Answer from the drawing. Dimensions are ordinates in mm from the lowest x, y and z of the part. Coordinates: 2 decimals unless noted, no trailing zeros. Loops run counter-clockwise (first coordinate to the right, second up) from the corner with the lowest first, then second, coordinate; pieces in that order, holes last.
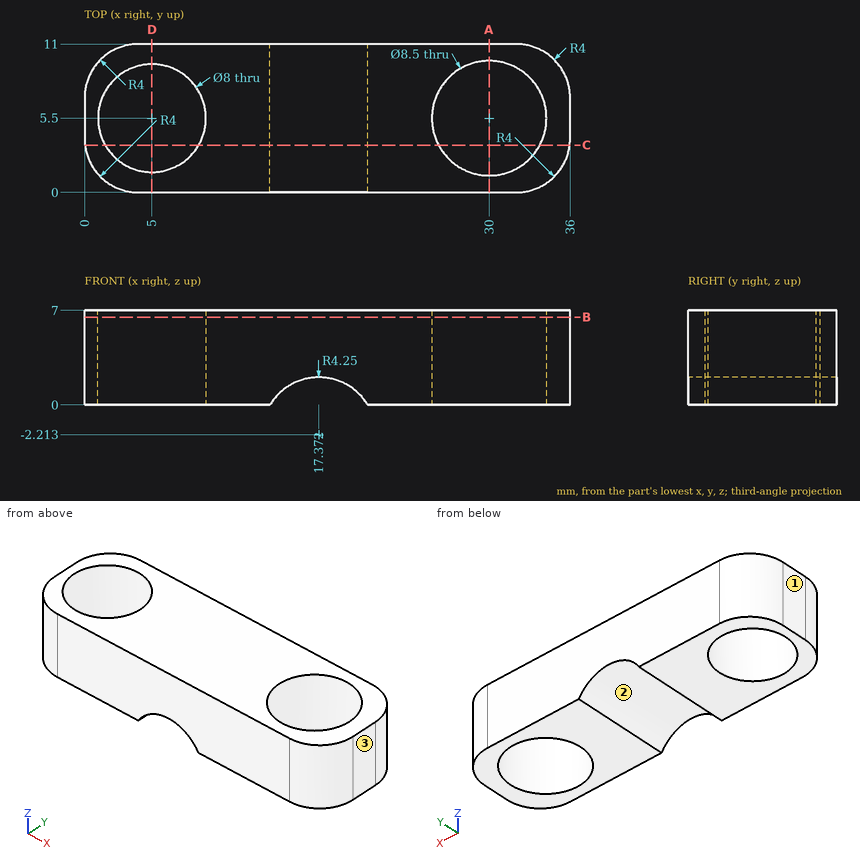
Item 1: Given pin 1 (4 mm diameter, centred on y = 1.5, z = 3.5, fed in from -X), flat-ended and moving along its own axis, determine where the tip first touches the part or whether it passes through.
Numbers:
pin 1: stops at x = 0.03
Item 2: Determine the mould class of the marked faces 1, 2 and 3 for opening direction X: released by +X, released by -X, zero draft, split by the parting line, or undercut.
Numbers:
face 1: released by -X
face 2: undercut
face 3: released by +X
Item 3: A cutting plane is placed at A-A on x = 30. Determine the outline of the cut face in (y, z).
Numbers:
outline: (0, 0) - (1.25, 0) - (1.25, 7) - (0, 7) - close; (9.75, 0) - (11, 0) - (11, 7) - (9.75, 7) - close
Item 4: A cutting plane is placed at B-B on z = 6.5. Determine the outline of the cut face in (x, y).
Numbers:
outline: (0, 4) arc R4 ccw to (4, 0) - (32, 0) arc R4 ccw to (36, 4) - (36, 7) arc R4 ccw to (32, 11) - (4, 11) arc R4 ccw to (0, 7) - close; hole circle Ø8 at (5, 5.5); hole circle Ø8.5 at (30, 5.5)
Item 5: Find the intervals of material crossed by line 1 along X through (y, z) = (5.75, 5); line 2 along Y through (x, z) = (30, 3.25); line 3 along Y through (x, z) = (5, 5), in increasing order.
Numbers:
line 1: x = 0 to 1.01, 8.99 to 25.76, 34.24 to 36
line 2: y = 0 to 1.25, 9.75 to 11
line 3: y = 0 to 1.5, 9.5 to 11
Item 6: A cutting plane is placed at D-D on x = 5. Determine the outline of the cut face in (y, z), then the cut area to 3 significant figures.
Numbers:
outline: (0, 0) - (1.5, 0) - (1.5, 7) - (0, 7) - close; (9.5, 0) - (11, 0) - (11, 7) - (9.5, 7) - close
area: 21.0 mm2
Item 7: A cutting plane is placed at C-C on y = 3.5. Determine the outline of the cut face in (x, z), then the cut area to 3 significant figures.
Numbers:
outline: (0.03, 0) - (1.54, 0) - (1.54, 7) - (0.03, 7) - close; (8.46, 0) - (13.74, 0) arc R4.25 cw to (21, 0) - (26.25, 0) - (26.25, 7) - (8.46, 7) - close; (33.75, 0) - (35.97, 0) - (35.97, 7) - (33.75, 7) - close
area: 140 mm2
